```python
from build123d import *

# Parameters (mm, degrees)
F0_W     = 80
F0_H     = 12.7
F1_DEPTH = 12.7
F3_D     = 3.2
F5_D     = 4.1
F7_D     = 10


with BuildPart() as f1:
    # F0 (on Top) → F1 (new body)
    with BuildSketch(Plane.XY):
        Rectangle(F0_W, F0_H)
    extrude(amount=F1_DEPTH)

    # F3 (through all)
    with Locations(Plane.XY.offset(12.7)):
        with Locations((-35, 0), (-20, 0)):
            Hole(F3_D / 2)

    # F5 (through all)
    with Locations(Plane.XY.offset(12.7)):
        with Locations((20, 0), (35, 0)):
            Hole(F5_D / 2)

    # F7 (through all)
    with Locations(Plane.XZ.offset(6.35)):
        with Locations((-3.75, 6.35), (3.75, 6.35)):
            Hole(F7_D / 2)


solid = f1.part
```
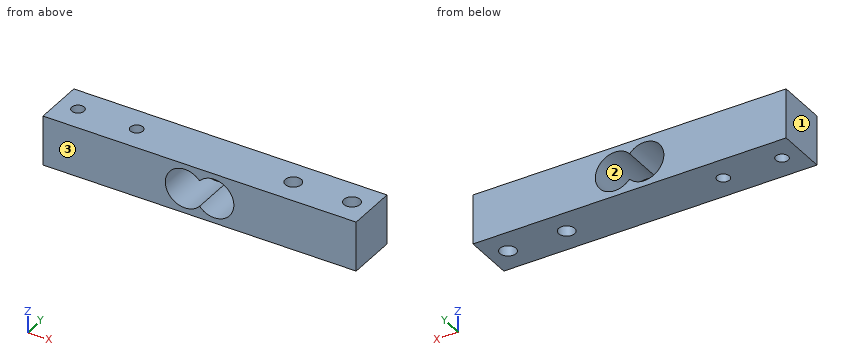
The listing builds one solid part. Answer for the finished solid, in the listing's coordinates (mm). Face numbers are marked on the shaded views. Give positions to 0.01 mm unless a question says otherwise; leave off trailing zeros. Loops run counter-clockwise (first coordinate to the right, second up) from the corner with the lowest first, then second, coordinate; pieces in that order, holes last. Notation, with made-up numbers: (-12.75, -10.5) - (35.25, -10.5) arc R22 cw to (35.25, -2.5) - close; hole circle Ø9 at (74.5, 78.25). An arc over 180 degrees is marked (long way). Return JSON: item names as keys, results as strings. Group by question number.
1. Find section B-B (x = 35). Write down the section's boundary in (y, z), then the cut area to 3 significant figures.
2. Find section A-A (z = 6.35). Write down the section's boundary in (x, y), then the cut area to 3 significant figures.
3. Given pin 1 Ø3.5 at (x, y) = (35, 0) entering from +Z (1 decimal); pin 2 Ø2 at (x, z) = (-7.5, 4.5) entering from +Y, each flat-ended and moving along its own axis, determine where each tip first touches the part or whether it passes through.
4. Find section C-C (y = 0). Write down the section's boundary in (x, z), then the cut area to 3 significant figures.
5. Straight lines are drawn through the part: line 1 (Y direction, x = 20, z = 9.75); line 2 (Z direction, x = -3.75, y = -2.75); line 3 (Y direction, x = -20, z = 8). For each, find the intervals that lie inside material, in ascending order. Write a range as [from, to].
6. Find section D-D (x = -20). Write down the section's boundary in (y, z).
7. Determine the mould class of the marked faces 1, 2 and 3 for opening direction X: pulls with the +X half, pulls with the -X half, needs draft (parallel to the pull), parting line crosses it, or undercut.
Verdict:
{
 "1": {"outline": "(-6.35, 0) - (-2.05, 0) - (-2.05, 12.7) - (-6.35, 12.7) - close; (2.05, 0) - (6.35, 0) - (6.35, 12.7) - (2.05, 12.7) - close", "area": "109 mm^2"},
 "2": {"outline": "(-40, -6.35) - (-8.75, -6.35) - (-8.75, 6.35) - (-40, 6.35) - close; (8.75, -6.35) - (40, -6.35) - (40, 6.35) - (8.75, 6.35) - close; hole circle Ø3.2 at (-35, 0); hole circle Ø3.2 at (-20, 0); hole circle Ø4.1 at (20, 0); hole circle Ø4.1 at (35, 0)", "area": "751 mm^2"},
 "3": {"pin 1": "passes through", "pin 2": "stops at y = 6.35"},
 "4": {"outline": "(-40, 0) - (-36.6, 0) - (-36.6, 12.7) - (-40, 12.7) - close; (-33.4, 0) - (-21.6, 0) - (-21.6, 12.7) - (-33.4, 12.7) - close; (-18.4, 0) - (17.95, 0) - (17.95, 12.7) - (-18.4, 12.7) - close; (22.05, 0) - (32.95, 0) - (32.95, 12.7) - (22.05, 12.7) - close; (37.05, 0) - (40, 0) - (40, 12.7) - (37.05, 12.7) - close; hole (0, 3.04) arc R5 ccw (long way) to (0, 9.66) arc R5 ccw (long way) to start", "area": "685 mm^2"},
 "5": {"line 1": "y = [-6.35, -2.05], [2.05, 6.35]", "line 2": "z = [0, 1.35], [11.35, 12.7]", "line 3": "y = [-6.35, -1.6], [1.6, 6.35]"},
 "6": {"outline": "(-6.35, 0) - (-1.6, 0) - (-1.6, 12.7) - (-6.35, 12.7) - close; (1.6, 0) - (6.35, 0) - (6.35, 12.7) - (1.6, 12.7) - close"},
 "7": {"face 1": "pulls with the -X half", "face 2": "undercut", "face 3": "needs draft"}
}
